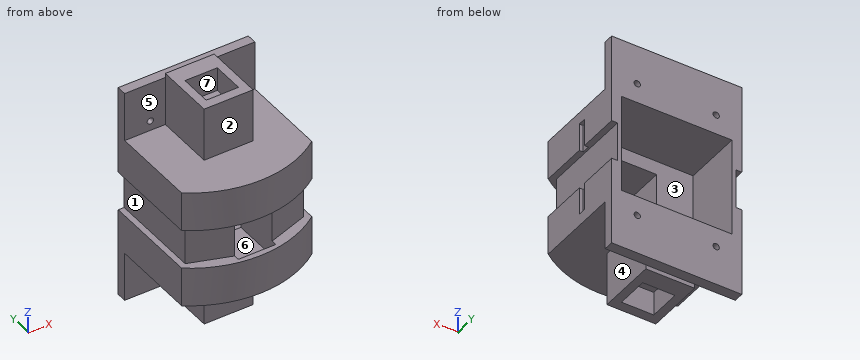
from build123d import *

# Parameters (mm, degrees)
BOSS_EXTRUDE1_DEPTH      = 30
BOSS_EXTRUDE1_DEPTH_BACK = 30
CUT_EXTRUDE1_DEPTH       = 18
CUT_EXTRUDE1_DEPTH_BACK  = 18
SKETCH3_W                = 21.854352608
SKETCH3_H                = 45
CUT_EXTRUDE2_DEPTH       = 99.234413522
SKETCH4_R                = 1.6
CUT_EXTRUDE3_DEPTH       = 84.366660003
SKETCH6_W                = 48
SKETCH6_H                = 4
CUT_EXTRUDE5_DEPTH       = 2
SKETCH9_W                = 22
SKETCH9_H                = 60
CUT_EXTRUDE7_DEPTH       = 84.366660003
SKETCH10_W               = 66
SKETCH10_H               = 25
SKETCH10_H_2             = 60
SKETCH10_W_2             = 19
SKETCH10_H_3             = 36
BOSS_EXTRUDE2_DEPTH      = 5
SKETCH11_R               = 1.6
CUT_EXTRUDE8_DEPTH       = 88.82938005
SKETCH13_W               = 24.8
SKETCH13_H               = 30
BOSS_EXTRUDE3_DEPTH      = 27.15
SKETCH14_W               = 16.4
SKETCH14_H               = 16.4
SKETCH14_W_2             = 16
SKETCH14_H_2             = 16
CUT_EXTRUDE9_DEPTH       = 12
SKETCH15_W               = 56
SKETCH15_H               = 50
CUT_EXTRUDE10_DEPTH      = 30
SKETCH16_W               = 19
SKETCH16_H               = 20
CUT_EXTRUDE11_DEPTH      = 45
CUT_EXTRUDE19_DEPTH      = 10
CUT_EXTRUDE19_DEPTH_BACK = 10


with BuildPart() as part:
    # Sketch1 → Boss-Extrude1 (new, two sides)
    with BuildSketch(Plane.XY) as boss_extrude1_sk:
        with BuildLine():
            Line((55, 0), (-55, 0))
            ThreePointArc((-55, 0), (0, -55), (55, 0))
        make_face()
    extrude(amount=BOSS_EXTRUDE1_DEPTH)
    extrude(boss_extrude1_sk.sketch, amount=-BOSS_EXTRUDE1_DEPTH_BACK)

    # Sketch2 → Cut-Extrude1 (cut, two sides)
    with BuildSketch(Plane.XY) as cut_extrude1_sk:
        Polygon((0, 0), (-9.5, 0), (-9.5, -52), (2.8860755, -52), (9.5, -52), (9.5, 0), align=None)
    extrude(amount=CUT_EXTRUDE1_DEPTH, mode=Mode.SUBTRACT)
    extrude(cut_extrude1_sk.sketch, amount=-CUT_EXTRUDE1_DEPTH_BACK, mode=Mode.SUBTRACT)

    # Sketch3 → Cut-Extrude2 (cut, through all)
    with BuildSketch(Plane.XY.offset(30)):
        with Locations((-43.927176304, -26.5)):
            Rectangle(SKETCH3_W, SKETCH3_H)
        with Locations((43.927176304, -26.5)):
            Rectangle(SKETCH3_W, SKETCH3_H)
    extrude(amount=-CUT_EXTRUDE2_DEPTH, mode=Mode.SUBTRACT)

    # Sketch4 → Cut-Extrude3 (cut, through all)
    with BuildSketch(Plane(origin=(0, 0, 0), x_dir=(1, 0, 0), z_dir=(0, 1, 0))):
        with Locations(Location((45, 20, 0), (0, 0, 270))):
            Circle(SKETCH4_R)
        with Locations(Location((45, -20, 0), (0, 0, 180))):
            Circle(SKETCH4_R)
        with Locations(Location((-45, -20, 0), (0, 0, 270))):
            Circle(SKETCH4_R)
        with Locations(Location((-45, 20, 0), (0, 0, 270))):
            Circle(SKETCH4_R)
    extrude(amount=-CUT_EXTRUDE3_DEPTH, mode=Mode.SUBTRACT)

    # Sketch6 → Cut-Extrude5 (cut)
    with BuildSketch(Plane(origin=(33, 0, 0), x_dir=(0, 0, -1), z_dir=(1, 0, 0))):
        with Locations((0, -18)):
            Rectangle(SKETCH6_W, SKETCH6_H)
    extrude(amount=-CUT_EXTRUDE5_DEPTH, mode=Mode.SUBTRACT)

    # Sketch9 → Cut-Extrude7 (cut, through all)
    with BuildSketch(Plane(origin=(0, 0, 0), x_dir=(1, 0, 0), z_dir=(0, 1, 0))):
        with Locations((-44, 0)):
            Rectangle(SKETCH9_W, SKETCH9_H)
        with Locations((44, 0)):
            Rectangle(SKETCH9_W, SKETCH9_H)
    extrude(amount=-CUT_EXTRUDE7_DEPTH, mode=Mode.SUBTRACT)

    # Sketch10 → Boss-Extrude2 (add)
    with BuildSketch(Plane(origin=(0, 0, 0), x_dir=(1, 0, 0), z_dir=(0, 1, 0))):
        with Locations((0, 42.5)):
            Rectangle(SKETCH10_W, SKETCH10_H)
        Rectangle(SKETCH10_W, SKETCH10_H_2)
        Rectangle(SKETCH10_W_2, SKETCH10_H_3, mode=Mode.SUBTRACT)
        with Locations((0, -42.5)):
            Rectangle(SKETCH10_W, SKETCH10_H)
    extrude(amount=BOSS_EXTRUDE2_DEPTH)

    # Sketch11 → Cut-Extrude8 (cut, through all)
    with BuildSketch(Plane(origin=(0, 5, 0), x_dir=(1, 0, 0), z_dir=(0, 1, 0))):
        with Locations(Location((-20, 35, 0), (0, 0, 270))):
            Circle(SKETCH11_R)
        with Locations(Location((20, 35, 0), (0, 0, 270))):
            Circle(SKETCH11_R)
        with Locations(Location((-20, -35, 0), (0, 0, 270))):
            Circle(SKETCH11_R)
        with Locations(Location((20, -35, 0), (0, 0, 270))):
            Circle(SKETCH11_R)
    extrude(amount=-CUT_EXTRUDE8_DEPTH, mode=Mode.SUBTRACT)

    # Sketch13 → Boss-Extrude3 (add)
    with BuildSketch(Plane(origin=(0, 0, -30), x_dir=(-1, 0, 0), z_dir=(0, 0, -1))):
        with Locations((0, -15)):
            Rectangle(SKETCH13_W, SKETCH13_H)
    boss_extrude3 = extrude(amount=BOSS_EXTRUDE3_DEPTH)

    # Sketch14 → Cut-Extrude9 (cut)
    with BuildSketch(Plane(origin=(0, 0, -57.15), x_dir=(-1, 0, 0), z_dir=(0, 0, -1))):
        with Locations((0, -17)):
            Rectangle(SKETCH14_W, SKETCH14_H)
        with Locations((0, -17)):
            Rectangle(SKETCH14_W_2, SKETCH14_H_2, mode=Mode.SUBTRACT)
        with Locations((0, -17)):
            Rectangle(SKETCH14_W_2, SKETCH14_H_2)
    cut_extrude9 = extrude(amount=-CUT_EXTRUDE9_DEPTH, mode=Mode.SUBTRACT)

    # Mirror2: Boss-Extrude3 across plane
    add(boss_extrude3.mirror(Plane(origin=(0, 0, 0), x_dir=(1, 0, 0), z_dir=(0, 0, -1))))

    # Mirror3: Cut-Extrude9 across plane
    add(cut_extrude9.mirror(Plane(origin=(0, 0, 0), x_dir=(1, 0, 0), z_dir=(0, 0, -1))), mode=Mode.SUBTRACT)

    # Sketch15 → Cut-Extrude10 (cut)
    with BuildSketch(Plane(origin=(0, 5, 0), x_dir=(1, 0, 0), z_dir=(0, 1, 0))):
        Rectangle(SKETCH15_W, SKETCH15_H)
    extrude(amount=-CUT_EXTRUDE10_DEPTH, mode=Mode.SUBTRACT)

    # Sketch16 → Cut-Extrude11 (cut)
    with BuildSketch(Plane(origin=(0, -52, 0), x_dir=(1, 0, 0), z_dir=(0, 1, 0))):
        Rectangle(SKETCH16_W, SKETCH16_H)
    extrude(amount=-CUT_EXTRUDE11_DEPTH, mode=Mode.SUBTRACT)

    # Sketch18 → Cut-Extrude19 (cut, two sides)
    with BuildSketch(Plane(origin=(0, 0, 0), x_dir=(-1, 0, 0), z_dir=(0, 0, -1))) as cut_extrude19_sk:
        Polygon((9.5, -49.173332923), (30, -42.194609519), (30, -41.173332923), (30, 5), (33, 5), (33, -41.173332923), (33, -54.173332923), (29.677482196, -54.173332923), (9.5, -54.173332923), align=None)
        Polygon((-30, -41.173332923), (-30, -42.194609519), (-9.5, -49.173332923), (-9.5, -54.173332923), (-29.677482196, -54.173332923), (-33, -54.173332923), (-33, -41.173332923), (-33, 5), (-30, 5), align=None)
    extrude(amount=CUT_EXTRUDE19_DEPTH, mode=Mode.SUBTRACT)
    extrude(cut_extrude19_sk.sketch, amount=-CUT_EXTRUDE19_DEPTH_BACK, mode=Mode.SUBTRACT)


solid = part.part
CAD build for the part. Positions are in the model's coordinates, mm. Face numbers are marked on the shaded views. A direction names the side the tool comes from. Round coordinates to 2 decimals unless told otherwise and drop trailing zeros. Loops run counter-clockwise (first coordinate to the right, second up) from the corner with the lowest first, then second, coordinate; pieces in that order, holes last.
(1) Which spindle directions (+Z, -Z, +X, -X, +Y, -Y) get a long thin tool onto all of the face, cutting with end or side? Do the marked faces 1, 2, 3 and 4. Say none if no direction does.
(2) Wall check: line 1 along X through (y, z) = (3.2, 35); line 2 along Z through (x, y) = (-7.5, -42.5); line 3 along Z through (x, y) = (10, -8). Give the ranges that are in metal, low to high.
(3) Two-plate mould, pull along Y, no slides. Class the marked faces 5, 6 and 7: +Y half, -Y half, draft (parallel to the pull), parting line (faces both ways), or undercut.
(4) Cut at A-A (z = -35). Give the cut face in (x, y).
(5) Drop flat-ended pins along their axis: pin 1 (1.2 mm diameter, centred on y = -18.5, z = 17.5, fed in from +X); pin 2 (15 mm diameter, centred on y = -13, z = -0.5, fed in from -X); pin 3 (13 mm diameter, centred on y = -20, z = 50.5, fed in from +X); pin 4 (13 mm diameter, centred on x = 3, y = -14, fed in from +Z). Give the stop position or say it passes through.
(6) Cut at D-D (z = -50). Give the cut face in (x, y).
(7) Cut at B-B (y = -39). Give the cut face in (x, z), plus the area to 3 significant figures.
Findings below:
1. face 1: -X, +Y, -Y
1. face 2: +Z, +X, -X, -Y
1. face 3: +Y
1. face 4: -Z, +X, -Y
2. line 1: x = -33 to -21.6, -18.4 to 18.4, 21.6 to 33
2. line 2: z = -30 to -18, 18 to 30
2. line 3: z = -57.15 to -25, 25 to 57.15
3. face 5: -Y half
3. face 6: draft
3. face 7: undercut
4. outline: (-33, 0) - (-21.6, 0) - (-21.6, 5) - (-33, 5) - close; (-18.4, 0) - (-12.4, 0) - (-12.4, -30) - (12.4, -30) - (12.4, 0) - (18.4, 0) - (18.4, 5) - (-18.4, 5) - close; (21.6, 0) - (33, 0) - (33, 5) - (21.6, 5) - close
5. pin 1: stops at x = 31
5. pin 2: stops at x = -30
5. pin 3: stops at x = 12.4
5. pin 4: stops at z = 57.15
6. outline: (-33, 0) - (-12.4, 0) - (-12.4, -30) - (12.4, -30) - (12.4, 0) - (33, 0) - (33, 5) - (-33, 5) - close; hole (-8.2, -25.2) - (8.2, -25.2) - (8.2, -8.8) - (-8.2, -8.8) - close
7. outline: (-33, -30) - (33, -30) - (33, -10) - (30, -10) - (30, 10) - (33, 10) - (33, 30) - (-33, 30) - (-33, 10) - (-30, 10) - (-30, -10) - (-33, -10) - close; hole (-9.5, -18) - (9.5, -18) - (9.5, 18) - (-9.5, 18) - close
7. area: 3,160 mm2
